from build123d import *

# Parameters (mm, degrees)
LINEAR_AUSTRAGEN_D_NN1_OUTLINE_R = 36
LINEAR_AUSTRAGEN_D_NN1_DEPTH     = 3
F_5_6_5_6_DURCHMESSER_BOHRUNG1_D = 5.6
KREISMUSTER1_COUNT               = 21


# Read off the part's stored shape, not the designer's step: Linear-Austragen-Dünn1
with BuildPart() as part:
    # Linear-Austragen-Dünn1 outline → Linear-Austragen-Dünn1 (new body)
    with BuildSketch(Plane(origin=(0, 0, 0), x_dir=(0, 0, -1), z_dir=(1, 0, 0))):
        with BuildLine():
            ThreePointArc((40.804878049, -3.995238094), (45, 0), (40.804878049, 3.995238094))
            ThreePointArc((40.804878049, 3.995238094), (40.542063875, 6.110732913), (40.169648908, 8.209708071))
            ThreePointArc((40.169648908, 8.209708071), (43.00077626, 13.263982848), (37.814414706, 15.845189821))
            ThreePointArc((37.814414706, 15.845189821), (36.939723584, 17.789233304), (35.96517018, 19.685185646))
            ThreePointArc((35.96517018, 19.685185646), (37.180744844, 25.349402613), (31.46397467, 26.287226897))
            ThreePointArc((31.46397467, 26.287226897), (30.055126745, 27.887082249), (28.565028251, 29.411548089))
            ThreePointArc((28.565028251, 29.411548089), (28.057041084, 35.182416711), (22.317822408, 34.393528504))
            ThreePointArc((22.317822408, 34.393528504), (20.5, 35.507041555), (18.626758206, 36.524565415))
            ThreePointArc((18.626758206, 36.524565415), (16.440346096, 41.889318689), (11.188633685, 39.44381417))
            ThreePointArc((11.188633685, 39.44381417), (9.123358292, 39.972044399), (7.033418953, 40.392214817))
            ThreePointArc((7.033418953, 40.392214817), (3.362854211, 44.874170873), (-0.934714242, 40.98934385))
            ThreePointArc((-0.934714242, 40.98934385), (-3.063933837, 40.885355684), (-5.18487044, 40.670838675))
            ThreePointArc((-5.18487044, 40.670838675), (-10.013442028, 43.871756048), (-12.975008707, 38.892790451))
            ThreePointArc((-12.975008707, 38.892790451), (-14.978981999, 38.165823694), (-16.942461341, 37.335680035))
            ThreePointArc((-16.942461341, 37.335680035), (-22.5, 38.97114317), (-23.862416708, 33.340441942))
            ThreePointArc((-23.862416708, 33.340441942), (-25.563081876, 32.055090781), (-27.194640201, 30.68308238))
            ThreePointArc((-27.194640201, 30.68308238), (-32.987334232, 30.6077732), (-32.629544266, 24.825648854))
            ThreePointArc((-32.629544266, 24.825648854), (-33.875789747, 23.096122381), (-35.030455938, 21.304158204))
            ThreePointArc((-35.030455938, 21.304158204), (-40.543599056, 19.52476826), (-38.497393623, 14.10498792))
            ThreePointArc((-38.497393623, 14.10498792), (-39.178485037, 12.084962151), (-39.753661936, 10.03226608))
            ThreePointArc((-39.753661936, 10.03226608), (-44.49738718, 6.706901977), (-40.944580614, 2.13103691))
            ThreePointArc((-40.944580614, 2.13103691), (-41, 0), (-40.944580614, -2.13103691))
            ThreePointArc((-40.944580614, -2.13103691), (-44.49738718, -6.706901977), (-39.753661936, -10.03226608))
            ThreePointArc((-39.753661936, -10.03226608), (-39.178485037, -12.084962151), (-38.497393623, -14.10498792))
            ThreePointArc((-38.497393623, -14.10498792), (-40.543599056, -19.52476826), (-35.030455938, -21.304158204))
            ThreePointArc((-35.030455938, -21.304158204), (-33.875789747, -23.096122381), (-32.629544266, -24.825648854))
            ThreePointArc((-32.629544266, -24.825648854), (-32.987334232, -30.6077732), (-27.194640201, -30.68308238))
            ThreePointArc((-27.194640201, -30.68308238), (-25.563081876, -32.055090781), (-23.862416708, -33.340441942))
            ThreePointArc((-23.862416708, -33.340441942), (-22.5, -38.97114317), (-16.942461341, -37.335680035))
            ThreePointArc((-16.942461341, -37.335680035), (-14.978981999, -38.165823694), (-12.975008707, -38.892790451))
            ThreePointArc((-12.975008707, -38.892790451), (-10.013442028, -43.871756048), (-5.18487044, -40.670838675))
            ThreePointArc((-5.18487044, -40.670838675), (-3.063933837, -40.885355684), (-0.934714242, -40.98934385))
            ThreePointArc((-0.934714242, -40.98934385), (3.362854211, -44.874170873), (7.033418953, -40.392214817))
            ThreePointArc((7.033418953, -40.392214817), (9.123358292, -39.972044399), (11.188633685, -39.44381417))
            ThreePointArc((11.188633685, -39.44381417), (16.440346096, -41.889318689), (18.626758206, -36.524565415))
            ThreePointArc((18.626758206, -36.524565415), (20.5, -35.507041555), (22.317822408, -34.393528504))
            ThreePointArc((22.317822408, -34.393528504), (28.057041084, -35.182416711), (28.565028251, -29.411548089))
            ThreePointArc((28.565028251, -29.411548089), (30.055126745, -27.887082249), (31.46397467, -26.287226897))
            ThreePointArc((31.46397467, -26.287226897), (37.180744844, -25.349402613), (35.96517018, -19.685185646))
            ThreePointArc((35.96517018, -19.685185646), (36.939723584, -17.789233304), (37.814414706, -15.845189821))
            ThreePointArc((37.814414706, -15.845189821), (43.00077626, -13.263982848), (40.169648908, -8.209708071))
            ThreePointArc((40.169648908, -8.209708071), (40.542063875, -6.110732913), (40.804878049, -3.995238094))
        make_face()
        Circle(LINEAR_AUSTRAGEN_D_NN1_OUTLINE_R, mode=Mode.SUBTRACT)
    extrude(amount=LINEAR_AUSTRAGEN_D_NN1_DEPTH)

    # Ø5.6 (5.6) Durchmesser Bohrung1 (through all)
    with Locations(Plane(origin=(3, 0, 0), x_dir=(0, 0, -1), z_dir=(1, 0, 0))):
        with Locations((41, 0)):
            f_5_6_5_6_durchmesser_bohrung1 = Hole(F_5_6_5_6_DURCHMESSER_BOHRUNG1_D / 2)

    # Kreismuster1: Ø5.6 (5.6) Durchmesser Bohrung1 ×21 about axis
    kreismuster1_axis = Axis((0, 0, 0), (1, 0, 0))
    for i in range(1, KREISMUSTER1_COUNT):
        add(f_5_6_5_6_durchmesser_bohrung1.rotate(kreismuster1_axis, i * 360 / KREISMUSTER1_COUNT), mode=Mode.SUBTRACT)


solid = part.part
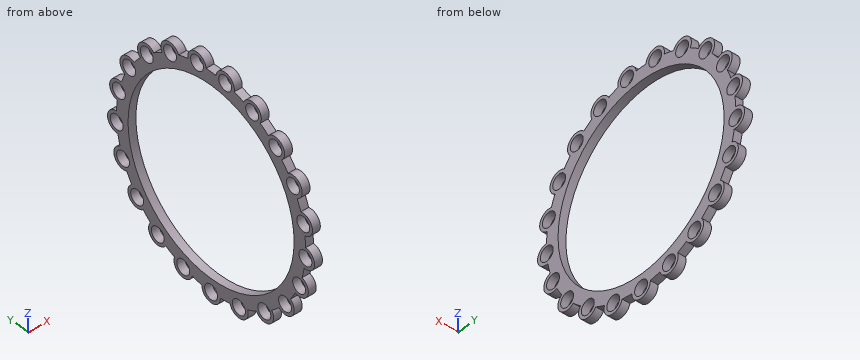
Part model, mm, in its own coordinate system. Coordinates: 2 decimals unless noted, no trailing zeros. Loops run counter-clockwise (first coordinate to the right, second up) from the corner with the lowest first, then second, coordinate; pieces in that order, holes last. Notation, with made-up numbers: (78, -16.5) - (93, -16.5) arc R13 cw to (93, 2.5) - close; hole circle Ø9 at (88, 88). An arc over 180 degrees is marked (long way). Write each question's results on one line, items separated by ' | '. Start each with the question number.
Q1. Slice it at D-D on z = 20.5. Give the cut face in (x, y).
Q2. Slice it at C-C on x = 1.9. Give the number of separate pieces and of enclosed holes in the cut face, and give its area (3 significant figures).
Q3. Drop a flat-ended pin along its axis: pin 1 Ø1.5 at (x, z) = (2, 34) entering from +Y. Give the stop position or say it passes through.
Q4. Probe line 1 along Y through (x, z) = (1.55, -29); line 2 along Y through (x, z) = (2.4, 29); line 3 along Z through (x, y) = (0.75, -14.5). List the from-to ranges inside material, lowest first.
Q5. Slice it at B-B on y = 0. Give the cut face in (x, z).
Q6. Slice it at A-A on z = -34. Give the cut face in (x, y).
Answer:
1) outline: (0, -39.51) - (3, -39.51) - (3, -38.31) - (0, -38.31) - close; (0, -32.71) - (3, -32.71) - (3, -29.59) - (0, -29.59) - close; (0, 29.59) - (3, 29.59) - (3, 32.71) - (0, 32.71) - close; (0, 38.31) - (3, 38.31) - (3, 39.51) - (0, 39.51) - close
2) separate pieces: 1 | enclosed holes: 22 | area: 1,230 mm2
3) pin 1: stops at y = 30.29
4) line 1: y = -34.1 to -30.01, -28.98 to -21.33, 21.33 to 28.98, 30.01 to 34.1 | line 2: y = -31.75 to -30.48, -25.29 to -21.33, 21.33 to 25.29, 30.48 to 31.75 | line 3: z = -42.37 to -40.6, -37.76 to -32.95, 32.95 to 39.22
5) outline: (0, -45) - (3, -45) - (3, -43.8) - (0, -43.8) - close; (0, -38.2) - (3, -38.2) - (3, -36) - (0, -36) - close; (0, 36) - (3, 36) - (3, 41) - (0, 41) - close
6) outline: (0, -27.09) - (3, -27.09) - (3, -25.89) - (0, -25.89) - close; (0, -20.3) - (3, -20.3) - (3, -11.83) - (0, -11.83) - close; (0, 11.83) - (3, 11.83) - (3, 20.3) - (0, 20.3) - close; (0, 25.89) - (3, 25.89) - (3, 27.09) - (0, 27.09) - close
